Can you work these out from the drawing? Everything is in mm from the part's minimum corner. Give positions to 0.01 mm unless a question says otherwise; leave off trailing zeros. Loops run counter-clockwise (first coordinate to the right, second up) from the corner with the lowest first, then second, coordinate; pieces in that order, holes last. Notation, with made-up numbers: (62.5, 45.25) -> (92.5, 45.25) arc R10 ccw to (92.5, 50.25) -> close; hole circle Ø4 at (71.25, 10). An arc over 180 degrees is marked (long way). Write item = value, one per line. Start each with the question number.
1) I want a section at B-B (y = 98.5). List the corners of the cut face in (x, z) for me.
2) I want a section at C-C (z = 29). List the corners of the cut face in (x, y) for me, and give its area (3 significant figures).
3) I'm going to push flat-ended pins straight in: pin 1 Ø1.5 at (x, z) = (1.5, 53) entering from -Y; pin 2 Ø1.5 at (x, y) = (1.5, 178) entering from +Z; pin 3 Ø1.5 at (x, z) = (1.5, 46) entering from +Y. Where does each tip first touch, or does it pass through?
4) I need wall thicknesses on probe 1 along Z at (x, y) = (1.9, 108.5); probe 2 along Y at (x, z) = (2.3, 26.5); probe 3 along Z at (x, y) = (2.25, 181). Which ranges of each line are inside material? Lowest first, please. Write a range as from..to.
5) I want a section at A-A (x = 2.25). List the corners of the cut face in (y, z) for me, and give its area (3 significant figures).
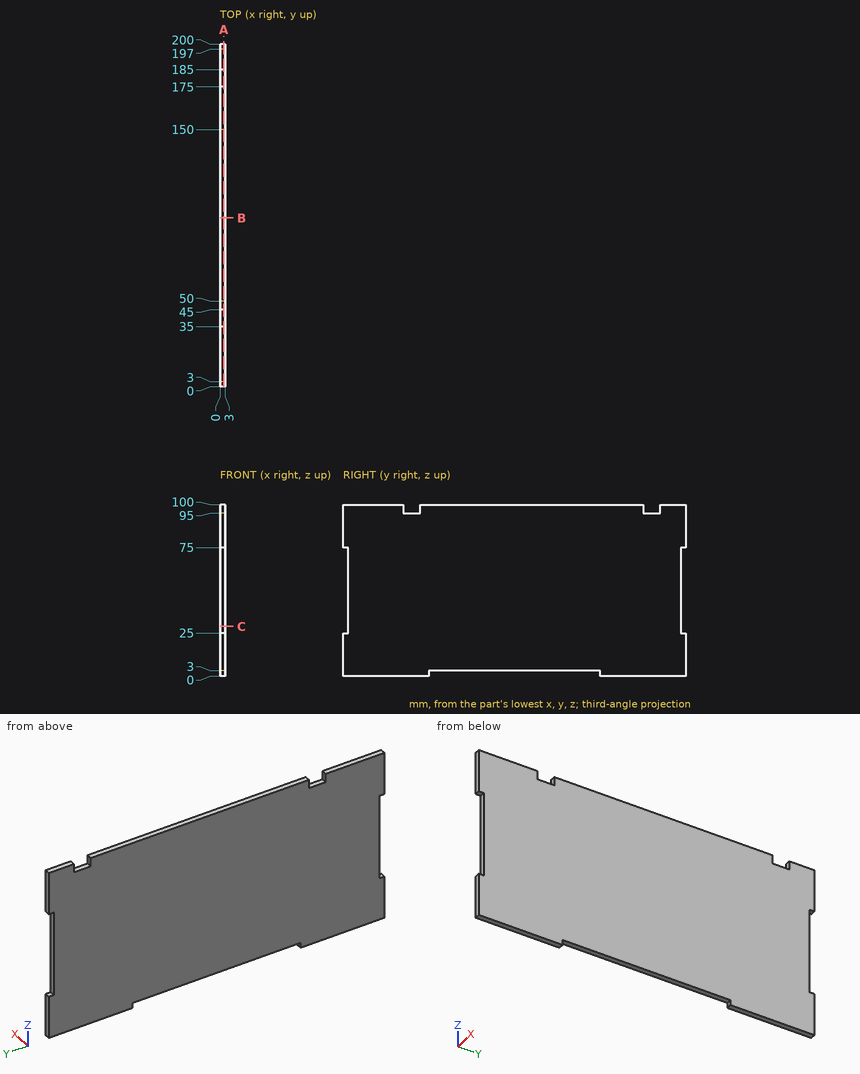
Answer list:
q1.outline = (0, 3) -> (3, 3) -> (3, 100) -> (0, 100) -> close
q2.outline = (0, 3) -> (3, 3) -> (3, 197) -> (0, 197) -> close
q2.area = 582 mm^2
q3.pin_1 = 3
q3.pin_2 = 95
q3.pin_3 = 197
q4.probe_1 = 3..100
q4.probe_2 = 3..197
q4.probe_3 = 0..95
q5.outline = (0, 0) -> (50, 0) -> (50, 3) -> (150, 3) -> (150, 0) -> (200, 0) -> (200, 25) -> (197, 25) -> (197, 75) -> (200, 75) -> (200, 100) -> (185, 100) -> (185, 95) -> (175, 95) -> (175, 100) -> (45, 100) -> (45, 95) -> (35, 95) -> (35, 100) -> (0, 100) -> (0, 75) -> (3, 75) -> (3, 25) -> (0, 25) -> close
q5.area = 19,300 mm^2
